Part print with two shaded views. Sizes in mm from the minimum x, y, z corner. Round coordinates to 2 decimals unless told otherwise and drop trailing zeros. Order: outer loops, then holes, each group sorted by start corner. A loop starts at its lowest first (then second) coordinate and runs counter-clockwise, first axis right, second up. Notation, with made-up numbers: (32.5, -23) - (79.5, -23) arc R13 ccw to (79.5, -3) - close; hole circle Ø8 at (32.25, 83). An arc over 180 degrees is marked (long way). Use one line per item in the form item = value.
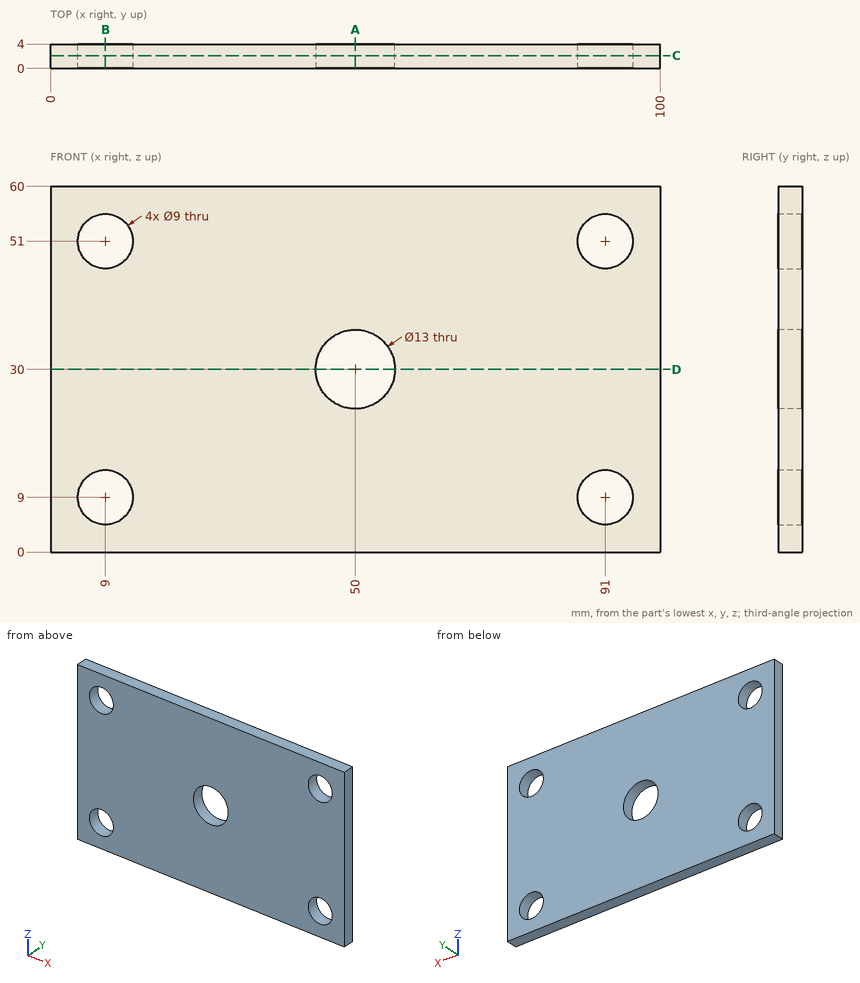
(1) Slice it at B-B on x = 9. Give the cut face in (y, z).
Report:
outline = (0, 0) - (4, 0) - (4, 4.5) - (0, 4.5) - close; (0, 13.5) - (4, 13.5) - (4, 46.5) - (0, 46.5) - close; (0, 55.5) - (4, 55.5) - (4, 60) - (0, 60) - close
(2) Probe probe 1 along Z at (x, y) = (9, 2.75); probe 2 along X at (y, z) = (1.75, 51); probe 3 along X at (y, z) = (2.2, 49). List the from-to ranges inside material, lowest first. Write a range as [from, to].
Report:
probe_1 = [0, 4.5], [13.5, 46.5], [55.5, 60]
probe_2 = [0, 4.5], [13.5, 86.5], [95.5, 100]
probe_3 = [0, 4.97], [13.03, 86.97], [95.03, 100]
(3) Pin check, flat tip, straight feed: pin 1 (8 mm diameter, centred on x = 50, z = 30, fed in from +Y). Stop position of the tip, or through.
Report:
pin_1 = through
(4) Slice it at A-A on x = 50. Give the cut face in (y, z), then the cut area to 3 significant figures.
Report:
outline = (0, 0) - (4, 0) - (4, 23.5) - (0, 23.5) - close; (0, 36.5) - (4, 36.5) - (4, 60) - (0, 60) - close
area = 188 mm2
(5) Slice it at C-C on y = 2.1. Give the cut face in (x, z), then the cut area to 3 significant figures.
Report:
outline = (0, 0) - (100, 0) - (100, 60) - (0, 60) - close; hole circle Ø9 at (9, 9); hole circle Ø9 at (9, 51); hole circle Ø13 at (50, 30); hole circle Ø9 at (91, 9); hole circle Ø9 at (91, 51)
area = 5,610 mm2
(6) Slice it at D-D on z = 30. Give the cut face in (x, y).
Report:
outline = (0, 0) - (43.5, 0) - (43.5, 4) - (0, 4) - close; (56.5, 0) - (100, 0) - (100, 4) - (56.5, 4) - close
